from build123d import *

# Parameters (mm, degrees)
BASE_FLANGE1_DEPTH = 50.8
SKETCH6_R          = 2.4892
CUT_EXTRUDE1_DEPTH = 63.217039467
SKETCH7_R          = 2.4892
CUT_EXTRUDE2_DEPTH = 63.217039467
FILLET1_R          = 3.175


# Read off the part's stored shape, not the designer's step: Base-Flange1
with BuildPart() as part:
    # Base-Flange1 outline → Base-Flange1 (new body)
    with BuildSketch(Plane.XY):
        with BuildLine():
            Line((0.8128, -1.5875), (25.4, -1.5875))
            Line((25.4, -1.5875), (25.4, 0))
            Line((25.4, 0), (0.8128, 0))
            ThreePointArc((0.8128, 0), (0.238063608, 0.238063608), (0, 0.8128))
            Line((0, 0.8128), (0, 25.4))
            Line((0, 25.4), (-1.5875, 25.4))
            Line((-1.5875, 25.4), (-1.5875, 0.8128))
            ThreePointArc((-1.5875, 0.8128), (-0.884468407, -0.884468407), (0.8128, -1.5875))
        make_face()
    extrude(amount=BASE_FLANGE1_DEPTH)

    # Sketch6 → Cut-Extrude1 (cut, through all)
    with BuildSketch(Plane(origin=(0, 0, 0), x_dir=(0, 0, -1), z_dir=(1, 0, 0))):
        with Locations((-44.45, 19.05)):
            Circle(SKETCH6_R)
        with Locations((-31.75, 19.05)):
            Circle(SKETCH6_R)
        with Locations((-19.05, 19.05)):
            Circle(SKETCH6_R)
        with Locations((-6.35, 19.05)):
            Circle(SKETCH6_R)
        with Locations((-6.35, 6.35)):
            Circle(SKETCH6_R)
        with Locations((-19.05, 6.35)):
            Circle(SKETCH6_R)
        with Locations((-31.75, 6.35)):
            Circle(SKETCH6_R)
        with Locations((-44.45, 6.35)):
            Circle(SKETCH6_R)
    extrude(amount=-CUT_EXTRUDE1_DEPTH, mode=Mode.SUBTRACT)

    # Sketch7 → Cut-Extrude2 (cut, through all)
    with BuildSketch(Plane(origin=(0, 0, 0), x_dir=(1, 0, 0), z_dir=(0, 1, 0))):
        with Locations(Location((19.05, -6.35, 0), (0, 0, 270))):
            Circle(SKETCH7_R)
        with Locations(Location((19.05, -19.05, 0), (0, 0, 270))):
            Circle(SKETCH7_R)
        with Locations(Location((6.35, -19.05, 0), (0, 0, 270))):
            Circle(SKETCH7_R)
        with Locations(Location((6.35, -6.35, 0), (0, 0, 270))):
            Circle(SKETCH7_R)
        with Locations(Location((19.05, -31.75, 0), (0, 0, 270))):
            Circle(SKETCH7_R)
        with Locations(Location((19.05, -44.45, 0), (0, 0, 270))):
            Circle(SKETCH7_R)
        with Locations(Location((6.35, -31.75, 0), (0, 0, 270))):
            Circle(SKETCH7_R)
        with Locations(Location((6.35, -44.45, 0), (0, 0, 270))):
            Circle(SKETCH7_R)
    extrude(amount=-CUT_EXTRUDE2_DEPTH, mode=Mode.SUBTRACT)

    # Fillet1
    fillet1_edges = [part.edges().sort_by_distance(p)[0] for p in [
        (-0.79375, 25.4, 50.8),
        (-0.79375, 25.4, 0),
        (25.4, -0.79375, 50.8),
        (25.4, -0.79375, 0),
    ]]
    fillet(fillet1_edges, radius=FILLET1_R)


solid = part.part
Read the model definition and answer for the solid it produces. Units are mm, in the model's axes. A direction names the side the tool comes from. Give positions to 0.01 mm unless a question says otherwise; leave off trailing zeros. Loops run counter-clockwise (first coordinate to the right, second up) from the corner with the lowest first, then second, coordinate; pieces in that order, holes last. Notation, with made-up numbers: (-24.5, -6.75) -> (19.5, -6.75) arc R25 cw to (19.5, 17.25) -> close; hole circle Ø10 at (3, 42.5). An arc over 180 degrees is marked (long way). Use a Markdown table: item, result.
Q1. Section A-A, the plane x = 6.35 is taken. Determine the outline of the cut face in (y, z), then the cut area to 3 significant figures.
Solved:
| item | result |
|---|---|
| outline | (-1.59, 0) -> (0, 0) -> (0, 3.86) -> (-1.59, 3.86) -> close; (-1.59, 8.84) -> (0, 8.84) -> (0, 16.56) -> (-1.59, 16.56) -> close; (-1.59, 21.54) -> (0, 21.54) -> (0, 29.26) -> (-1.59, 29.26) -> close; (-1.59, 34.24) -> (0, 34.24) -> (0, 41.96) -> (-1.59, 41.96) -> close; (-1.59, 46.94) -> (0, 46.94) -> (0, 50.8) -> (-1.59, 50.8) -> close |
| area | 49.0 mm^2 |
Q2. Section D-D, the plane z = 33 is taken. Determine the outline of the cut face in (x, y), then the cut area to 3 significant figures.
Solved:
| item | result |
|---|---|
| outline | (-1.59, 0.81) arc R2.4 ccw to (0.81, -1.59) -> (4.2, -1.59) -> (4.2, 0) -> (0.81, 0) arc R0.81 cw to (0, 0.81) -> (0, 4.2) -> (-1.59, 4.2) -> close; (-1.59, 8.5) -> (0, 8.5) -> (0, 16.9) -> (-1.59, 16.9) -> close; (-1.59, 21.2) -> (0, 21.2) -> (0, 25.4) -> (-1.59, 25.4) -> close; (8.5, -1.59) -> (16.9, -1.59) -> (16.9, 0) -> (8.5, 0) -> close; (21.2, -1.59) -> (25.4, -1.59) -> (25.4, 0) -> (21.2, 0) -> close |
| area | 54.7 mm^2 |
Q3. Each of these flat-tipped pins is pushed along its axis until it touches: pin 1 (8 mm diameter, centred on x = 19.05, z = 44.45, fed in from +Y); pin 2 (5.5 mm diameter, centred on x = 19.05, z = 19.05, fed in from -Y); pin 3 (5 mm diameter, centred on y = 7, z = 12.5, fed in from +X); pin 4 (3 mm diameter, centred on x = 6.35, z = 19.05, fed in from -Y). Where does it stop, or does it pass through?
Solved:
| item | result |
|---|---|
| pin 1 | stops at y = 0 |
| pin 2 | stops at y = -1.59 |
| pin 3 | stops at x = 0 |
| pin 4 | passes through |
Q4. Determine the mould class of faces 3 (the face through (18.1, -0.78, 46.75)), 4 (the face through (-1, 25.4, 25)), 5 (the face through (-1.588, 13, 25)) for opening direction X: pulls with the +X half, pulls with the -X half, needs draft (parallel to the pull), parting line crosses it, or undercut.
Solved:
| item | result |
|---|---|
| face 3 | undercut |
| face 4 | needs draft |
| face 5 | pulls with the -X half |
Q5. A tool of negligible diameter and unlimited length cuts with its end or side. For faces 1 (the face through (-0.783, 4.142, 5.201)), 2 (the face through (13, 0, 25)), from which of +Z, -Z, +X, -X, +Y, -Y can it reach the whole face along a straight path? Write none if from no direction.
Solved:
| item | result |
|---|---|
| face 1 | +X, -X |
| face 2 | +Z, -Z, +X, +Y |
Q6. Section C-C, the plane z = 19.05 is taken. Determine the outline of the cut face in (x, y), then the cut area to 3 significant figures.
Solved:
| item | result |
|---|---|
| outline | (-1.59, 0.81) arc R2.4 ccw to (0.81, -1.59) -> (3.86, -1.59) -> (3.86, 0) -> (0.81, 0) arc R0.81 cw to (0, 0.81) -> (0, 3.86) -> (-1.59, 3.86) -> close; (-1.59, 8.84) -> (0, 8.84) -> (0, 16.56) -> (-1.59, 16.56) -> close; (-1.59, 21.54) -> (0, 21.54) -> (0, 25.4) -> (-1.59, 25.4) -> close; (8.84, -1.59) -> (16.56, -1.59) -> (16.56, 0) -> (8.84, 0) -> close; (21.54, -1.59) -> (25.4, -1.59) -> (25.4, 0) -> (21.54, 0) -> close |
| area | 50.5 mm^2 |
Q7. Find the intervals of material crossed by line 1 along X through (y, z) = (-0.3, 31.75); line 2 along X through (y, z) = (-0.8, 19.05); line 3 along Y through (x, z) = (-0.7, 31.75), in increasing order.
Solved:
| item | result |
|---|---|
| line 1 | x = -1.31 to 3.86, 8.84 to 16.56, 21.54 to 25.4 |
| line 2 | x = -0.96 to 3.86, 8.84 to 16.56, 21.54 to 25.4 |
| line 3 | y = -1.05 to 3.86, 8.84 to 16.56, 21.54 to 25.4 |
